from build123d import *

# Parameters (mm, degrees)
SKETCH1_R           = 3.2
SKETCH1_R_2         = 1.1303
BOSS_EXTRUDE1_DEPTH = 10
SKETCH2_W           = 5.5
SKETCH2_H           = 38
CUT_EXTRUDE1_DEPTH  = 2
FILLET3_R           = 0.5
SKETCH5_R           = 5
CUT_EXTRUDE2_DEPTH  = 4
FILLET1_R           = 4
SKETCH4_R           = 1.397
BOSS_EXTRUDE2_DEPTH = 5.08
CUT_EXTRUDE3_DEPTH  = 2.54
FILLET5_R           = 3.175
FILLET4_R           = 1


with BuildPart() as part:
    # Sketch1 → Boss-Extrude1 (new body)
    with BuildSketch(Plane(origin=(0, 0, 0), x_dir=(1, 0, 0), z_dir=(0, 1, 0))):
        Polygon((-17, 22.225), (-5, 22.225), (-5, 9.525), (8, 9.525), (8, -9.525), (-5, -9.525), (-5, -22.225), (-17, -22.225), align=None)
        with Locations(Location((0, 0, 0), (0, 0, 270))):
            Circle(SKETCH1_R, mode=Mode.SUBTRACT)
        with Locations(Location((-11, 14.2875, 0), (0, 0, 270))):
            Circle(SKETCH1_R_2, mode=Mode.SUBTRACT)
        with Locations(Location((-11, -14.2875, 0), (0, 0, 90))):
            Circle(SKETCH1_R_2, mode=Mode.SUBTRACT)
    extrude(amount=BOSS_EXTRUDE1_DEPTH)

    # Sketch2 → Cut-Extrude1 (cut)
    with BuildSketch(Plane(origin=(0, 10, 0), x_dir=(1, 0, 0), z_dir=(0, 1, 0))):
        with Locations((-11, 0)):
            Rectangle(SKETCH2_W, SKETCH2_H)
    extrude(amount=-CUT_EXTRUDE1_DEPTH, mode=Mode.SUBTRACT)

    # Fillet3
    fillet3_edges = [part.edges().sort_by_distance(p)[0] for p in [
        (-13.75, 9, 19),
        (-13.75, 9, -19),
        (-8.25, 9, -19),
        (-8.25, 9, 19),
    ]]
    fillet(fillet3_edges, radius=FILLET3_R)

    # Sketch5 → Cut-Extrude2 (cut)
    with BuildSketch(Plane(origin=(0, 10, 0), x_dir=(1, 0, 0), z_dir=(0, 1, 0))):
        with Locations(Location((0, 0, 0), (0, 0, 270))):
            Circle(SKETCH5_R)
    extrude(amount=-CUT_EXTRUDE2_DEPTH, mode=Mode.SUBTRACT)

    # Fillet1
    fillet1_edges = [part.edges().sort_by_distance(p)[0] for p in [
        (-17, 5, 22.225),
        (-17, 5, -22.225),
        (-5, 5, -22.225),
        (-5, 5, -9.525),
        (8, 5, -9.525),
        (8, 5, 9.525),
        (-5, 5, 9.525),
        (-5, 5, 22.225),
    ]]
    fillet(fillet1_edges, radius=FILLET1_R)

    # Sketch4 → Boss-Extrude2 (add)
    with BuildSketch(Plane.ZY.offset(17)):
        Polygon((-4.7625, 10), (4.7625, 10), (4.7625, 22.2875), (14.2875, 22.2875), (14.2875, 0), (-14.2875, 0), (-14.2875, 22.2875), (-4.7625, 22.2875), align=None)
        with Locations((-9.525, 17.525)):
            Circle(SKETCH4_R, mode=Mode.SUBTRACT)
        with Locations((9.525, 17.525)):
            Circle(SKETCH4_R, mode=Mode.SUBTRACT)
    extrude(amount=BOSS_EXTRUDE2_DEPTH)

    # Sketch6 → Cut-Extrude3 (cut)
    with BuildSketch(Plane(origin=(-17, 0, 0), x_dir=(0, 0, -1), z_dir=(1, 0, 0))):
        Polygon((-6.35, 15.691912895), (-6.35, 19.358087105), (-9.525, 21.191174209), (-12.7, 19.358087105), (-12.7, 15.691912895), (-9.525, 13.858825791), align=None)
    cut_extrude3 = extrude(amount=-CUT_EXTRUDE3_DEPTH, mode=Mode.SUBTRACT)

    # Mirror1: Cut-Extrude3 across plane
    add(cut_extrude3.mirror(Plane.XY), mode=Mode.SUBTRACT)

    # Fillet5
    fillet5_edges = [part.edges().sort_by_distance(p)[0] for p in [
        (-19.54, 22.2875, 14.2875),
        (-19.54, 22.2875, 4.7625),
        (-19.54, 10, 4.7625),
        (-19.54, 10, -4.7625),
        (-19.54, 22.2875, -4.7625),
        (-19.54, 22.2875, -14.2875),
    ]]
    fillet(fillet5_edges, radius=FILLET5_R)

    # Fillet4
    fillet4_edges = [part.edges().sort_by_distance(p)[0] for p in [
        (-22.08, 9.55625, 14.2875),
        (-22.08, 10, 0),
        (-22.08, 16.14375, 4.7625),
        (-22.08, 16.14375, -4.7625),
        (-22.08, 22.2875, 9.525),
        (-22.08, 22.2875, -9.525),
        (-22.08, 9.55625, -14.2875),
        (-22.08, 21.35756403, -13.35756403),
        (-22.08, 21.35756403, -5.69243597),
        (-22.08, 21.35756403, 5.69243597),
        (-22.08, 21.35756403, 13.35756403),
        (-22.08, 10.92993597, 3.83256403),
        (-22.08, 10.92993597, -3.83256403),
    ]]
    fillet(fillet4_edges, radius=FILLET4_R)


solid = part.part
Could you check a few things on this model? Use its own coordinates, in mm. A direction names the side the tool comes from. Coordinates: 2 decimals unless noted, no trailing zeros. Order: outer loops, then holes, each group sorted by start corner. A loop starts at its lowest first (then second) coordinate and runs counter-clockwise, first axis right, second up. Notation, with made-up numbers: (60.25, 5.5) - (68.25, 5.5) arc R14 cw to (68.25, 27.5) - close; hole circle Ø10 at (-29.75, 57). An arc over 180 degrees is marked (long way). Answer in a Markdown table with one row per item. Add a question column.
(1) If we section it at A-A, the plane z = -17: Please give me the cut outline in (x, y).
(2) On a 3-axis mill with a long thin cutter (end or side, diameter ignored), from which of +Z, -Z, +X, -X, +Y, -Y can I reach the whole of each face in a straight line? I mean faces 5 (the face through (-17, 13, -9)), 6 (the face through (-19.1, 10.9, -3.8)), 7 (the face through (-21.779, 9.715, 0.022)). Say none if no direction works.
(3) Will these pins go through, and if not, where does the flat tip stop? pin 1 (3.5 mm diameter, centred on y = 17.525, z = -9.525, fed in from +X); pin 2 (1.3 mm diameter, centred on x = -18, y = 16.5, fed in from +Z); pin 3 (1.5 mm diameter, centred on y = 9, z = 8, fed in from +X); pin 4 (1 mm diameter, centred on x = -8, z = -7, fed in from -Y).
(4) If we section it at C-C, the plane y = 4.25: Please give me the cut outline in (x, z) (1 decimal).
(5) If we section it at D-D, the plane x = -4.5: Please give me the cut outline in (y, z), then the cut area to 3 significant figures.
(6) I need wall thicknesses on L1, parallel to X at y = 2.7, z = 0; L2, parallel to X at y = 6.75, z = 18.5; L3, parallel to X at y = 14.5, z = -7.5. Which ranges of each line are inside material? Lowest first, please.
(7) If we section it at B-B, the plane x = 0: Please give me the cut outline in (y, z) (3 decimals), then the cut area to 3 significant figures.
(8) If we mould it in two halves opening along X, with no side actions, what happens to faces 1 (the face through (-21.78, 16.1, -5.05)), 2 (the face through (-8.25, 9, 0)), 3 (the face through (-11, 5, 22.225)), 4 (the face through (-11.764, 3.944, 15.121))? For each: released by +X, released by -X, zero draft, split by the parting line, or undercut.
Results are:
| question | item | result |
|---|---|---|
| 1 | outline | (-17, 0) - (-5, 0) - (-5, 10) - (-8.25, 10) - (-8.25, 8) - (-13.75, 8) - (-13.75, 10) - (-17, 10) - close |
| 2 | face 5 | +Z, -Z, +X, +Y |
| 2 | face 6 | +X, -X, +Y |
| 2 | face 7 | -X, +Y |
| 3 | pin 1 | stops at x = -19.54 |
| 3 | pin 2 | stops at z = 14.29 |
| 3 | pin 3 | stops at x = 7.61 |
| 3 | pin 4 | stops at y = 0 |
| 4 | outline | (-22.1, -13.3) arc R1 ccw to (-21.1, -14.3) - (-17, -14.3) - (-17, -18.2) arc R4 ccw to (-13, -22.2) - (-9, -22.2) arc R4 ccw to (-5, -18.2) - (-5, -13.5) arc R4 cw to (-1, -9.5) - (4, -9.5) arc R4 ccw to (8, -5.5) - (8, 5.5) arc R4 ccw to (4, 9.5) - (-1, 9.5) arc R4 cw to (-5, 13.5) - (-5, 18.2) arc R4 ccw to (-9, 22.2) - (-13, 22.2) arc R4 ccw to (-17, 18.2) - (-17, 14.3) - (-21.1, 14.3) arc R1 ccw to (-22.1, 13.3) - close; hole circle Ø2.3 at (-11, -14.3); hole circle Ø2.3 at (-11, 14.3); hole circle Ø6.4 at (0, 0) |
| 5 | outline | (0, -11.59) - (10, -11.59) - (10, -2.18) - (6, -2.18) - (6, 2.18) - (10, 2.18) - (10, 11.59) - (0, 11.59) - close |
| 5 | area | 214 mm2 |
| 6 | L1 | x = -22.08 to -3.2, 3.2 to 8 |
| 6 | L2 | x = -16.99 to -5.01 |
| 6 | L3 | x = -22.08 to -17 |
| 7 | outline | (0, -9.525) - (10, -9.525) - (10, -5) - (6, -5) - (6, -3.2) - (0, -3.2) - close; (0, 3.2) - (6, 3.2) - (6, 5) - (10, 5) - (10, 9.525) - (0, 9.525) - close |
| 7 | area | 112 mm2 |
| 8 | face 1 | released by -X |
| 8 | face 2 | undercut |
| 8 | face 3 | zero draft |
| 8 | face 4 | undercut |
